from build123d import *

# Parameters (mm, degrees)
BOSS_EXTRU_1_DEPTH      = 11.3
ESQUISSE2_W             = 8.6
ESQUISSE2_H             = 11.3
BOSS_EXTRU_2_DEPTH      = 1
ESQUISSE8_W             = 11.3
ESQUISSE8_H             = 1
BOSS_EXTRU_5_DEPTH      = 10
ESQUISSE9_W             = 2
ESQUISSE9_H             = 11.3
BOSS_EXTRU_6_DEPTH      = 7.8
ESQUISSE10_W            = 11.3
ESQUISSE10_H            = 2
BOSS_EXTRU_7_DEPTH      = 39.7
ESQUISSE11_W            = 2
ESQUISSE11_H            = 11.3
BOSS_EXTRU_8_DEPTH      = 11.3
ESQUISSE12_W            = 2
ESQUISSE12_H            = 11.3
BOSS_EXTRU_9_DEPTH      = 11.3
BOSS_EXTRU_10_DEPTH     = 11.3
ESQUISSE14_W            = 1
ESQUISSE14_H            = 11.3
BOSS_EXTRU_11_DEPTH     = 5.8
ESQUISSE16_W            = 11.3
ESQUISSE16_H            = 6.8
ENL_V_MAT_EXTRU_1_DEPTH = 1
ESQUISSE19_R            = 2
ENL_V_MAT_EXTRU_3_DEPTH = 10


with BuildPart() as part:
    # Esquisse1 → Boss.-Extru.1 (new body)
    with BuildSketch(Plane.XY):
        Polygon((-20.6, 1), (-20.6, 0), (-24.6, 0), (-24.6, 13.6), (0, 13.6), (0, 0), (-4, 0), (-4, 1), (-1, 1), (-1, 12.6), (-23.6, 12.6), (-23.6, 1), align=None)
    extrude(amount=BOSS_EXTRU_1_DEPTH)

    # Esquisse2 → Boss.-Extru.2 (add)
    with BuildSketch(Plane(origin=(0, 13.6, 0), x_dir=(1, 0, 0), z_dir=(0, 1, 0))):
        with Locations((-12.3, -5.65)):
            Rectangle(ESQUISSE2_W, ESQUISSE2_H)
    extrude(amount=BOSS_EXTRU_2_DEPTH)

    # Esquisse8 → Boss.-Extru.5 (add)
    with BuildSketch(Plane(origin=(-8, 0, 0), x_dir=(0, 0, -1), z_dir=(1, 0, 0))):
        with Locations((-5.65, 14.1)):
            Rectangle(ESQUISSE8_W, ESQUISSE8_H)
    extrude(amount=BOSS_EXTRU_5_DEPTH)

    # Esquisse9 → Boss.-Extru.6 (add)
    with BuildSketch(Plane.XZ.offset(-13.6)):
        with Locations((1, 5.65)):
            Rectangle(ESQUISSE9_W, ESQUISSE9_H)
    extrude(amount=BOSS_EXTRU_6_DEPTH)

    # Esquisse10 → Boss.-Extru.7 (add)
    with BuildSketch(Plane(origin=(2, 0, 0), x_dir=(0, 0, -1), z_dir=(1, 0, 0))):
        with Locations((-5.65, 6.8)):
            Rectangle(ESQUISSE10_W, ESQUISSE10_H)
    extrude(amount=BOSS_EXTRU_7_DEPTH)

    # Esquisse11 → Boss.-Extru.8 (add)
    with BuildSketch(Plane.XZ.offset(-5.8)):
        with Locations((40.7, 5.65)):
            Rectangle(ESQUISSE11_W, ESQUISSE11_H)
    extrude(amount=BOSS_EXTRU_8_DEPTH)

    # Esquisse12 → Boss.-Extru.9 (add)
    with BuildSketch(Plane(origin=(0, 7.8, 0), x_dir=(1, 0, 0), z_dir=(0, 1, 0))):
        with Locations((40.7, -5.65)):
            Rectangle(ESQUISSE12_W, ESQUISSE12_H)
    extrude(amount=BOSS_EXTRU_9_DEPTH)

    # Esquisse13 → Boss.-Extru.10 (add)
    with BuildSketch(Plane.XY.offset(11.3)):
        Polygon((-16.6, 14.6), (-25.6, 14.6), (-25.6, 0), (-24.6, 0), (-24.6, 13.6), (-16.6, 13.6), align=None)
    extrude(amount=-BOSS_EXTRU_10_DEPTH)

    # Esquisse14 → Boss.-Extru.11 (add)
    with BuildSketch(Plane.XZ.offset(-5.8)):
        with Locations((0.5, 5.65)):
            Rectangle(ESQUISSE14_W, ESQUISSE14_H)
    extrude(amount=BOSS_EXTRU_11_DEPTH)

    # Esquisse16 → Enlèv. mat.-Extru.1 (cut)
    with BuildSketch(Plane(origin=(2, 0, 0), x_dir=(0, 0, -1), z_dir=(1, 0, 0))):
        with Locations((-5.65, 11.2)):
            Rectangle(ESQUISSE16_W, ESQUISSE16_H)
    extrude(amount=-ENL_V_MAT_EXTRU_1_DEPTH, mode=Mode.SUBTRACT)

    # Esquisse19 → Enlèv. mat.-Extru.3 (cut)
    with BuildSketch(Plane(origin=(41.7, 0, 0), x_dir=(0, 0, -1), z_dir=(1, 0, 0))):
        with Locations((-5.65, 13.45)):
            Circle(ESQUISSE19_R)
        with Locations((-5.65, 2.15)):
            Circle(ESQUISSE19_R)
    extrude(amount=-ENL_V_MAT_EXTRU_3_DEPTH, mode=Mode.SUBTRACT)


solid = part.part
Build history of the part. All positions in model axes, mm. A direction names the side the tool comes from. Coordinates: 2 decimals unless noted, no trailing zeros. Order: outer loops, then holes, each group sorted by start corner. A loop starts at its lowest first (then second) coordinate and runs counter-clockwise, first axis right, second up. Notation, with made-up numbers: (-3.5, 63.25) -> (11.5, 63.25) arc R20 cw to (11.5, 71.25) -> close; hole circle Ø6 at (-13.75, -3). An arc over 180 degrees is marked (long way). One line per item, written item: value.
(1) Tool access for faces 1 (the cylindrical face through (40.714, 1.384, 3.803)), 2 (the flat face through (-2, 0, 6)), 3 (the flat face through (20, 5.8, 6)), 4 (the flat face through (21, 7.8, 6)): list every direction of +Z, -Z, +X, -X, +Y, -Y with a clear straight run to the whole face (end or side of a thin tool).
Checked values:
face 1: +X
face 2: +Z, -Z, -X, -Y
face 3: +Z, -Z, -Y
face 4: +Z, -Z, +Y
(2) Slice it at C-C, the plane y = 13.45. List the corners of the cut face in (x, z), plus the area to 3 significant figures.
Checked values:
outline: (-25.6, 0) -> (1, 0) -> (1, 11.3) -> (-25.6, 11.3) -> close; (39.7, 0) -> (41.7, 0) -> (41.7, 3.65) -> (39.7, 3.65) -> close; (39.7, 7.65) -> (41.7, 7.65) -> (41.7, 11.3) -> (39.7, 11.3) -> close
area: 315 mm2
(3) Mould opens along X. For faces 5 (the flat face through (-22, 1, 6)), 6 (the flat face through (41.7, 7, 6)), 7 (the flat face through (-23, 0, 6)) say: pulls with the +X half, pulls with the -X half, needs draft (parallel to the pull), parting line crosses it, or undercut.
Checked values:
face 5: undercut
face 6: pulls with the +X half
face 7: needs draft
(4) Drop flat-ended pins along their axis: pin 1 Ø5.5 at (x, z) = (-23, 3) entering from -Y; pin 2 Ø4 at (x, z) = (-0.5, 3) entering from +Y; pin 3 Ø5.5 at (x, z) = (16.5, 7) entering from +Y. Give the stop position or say it passes through.
Checked values:
pin 1: y = 0
pin 2: y = 14.6
pin 3: y = 7.8
(5) Slice it at B-B, the plane y = 7. List the corners of the cut face in (x, z), plus the area to 3 significant figures.
Checked values:
outline: (-25.6, 0) -> (-23.6, 0) -> (-23.6, 11.3) -> (-25.6, 11.3) -> close; (-1, 0) -> (41.7, 0) -> (41.7, 11.3) -> (-1, 11.3) -> close
area: 505 mm2
(6) Slice it at A-A, the plane z = 5.65. List the corners of the cut face in (x, y), plus the area to 3 significant figures.
Checked values:
outline: (-25.6, 0) -> (-20.6, 0) -> (-20.6, 1) -> (-23.6, 1) -> (-23.6, 12.6) -> (-1, 12.6) -> (-1, 1) -> (-4, 1) -> (-4, 0) -> (1, 0) -> (1, 5.8) -> (39.7, 5.8) -> (39.7, 4.15) -> (41.7, 4.15) -> (41.7, 11.45) -> (39.7, 11.45) -> (39.7, 7.8) -> (1, 7.8) -> (1, 14.6) -> (-25.6, 14.6) -> close; (39.7, -5.5) -> (41.7, -5.5) -> (41.7, 0.15) -> (39.7, 0.15) -> close; (39.7, 15.45) -> (41.7, 15.45) -> (41.7, 19.1) -> (39.7, 19.1) -> close
area: 220 mm2
(7) Probe line 1 (X direction, y = 4.5, z = 9.5); line 2 (Y direction, x = 41.3, z = 5.65); line 3 (X direction, y = 13.5, z = 9.75). List the from-to ranges inside material, lowest first. Write a range as [from, to].
Checked values:
line 1: [-25.6, -23.6], [-1, 1], [39.7, 41.7]
line 2: [-5.5, 0.15], [4.15, 11.45], [15.45, 19.1]
line 3: [-25.6, 1], [39.7, 41.7]
(8) Slice it at D-D, the plane y = 2.15. List the corners of the cut face in (x, z), plus the area to 3 significant figures.
Checked values:
outline: (-25.6, 0) -> (-23.6, 0) -> (-23.6, 11.3) -> (-25.6, 11.3) -> close; (-1, 0) -> (1, 0) -> (1, 11.3) -> (-1, 11.3) -> close; (39.7, 0) -> (41.7, 0) -> (41.7, 3.65) -> (39.7, 3.65) -> close; (39.7, 7.65) -> (41.7, 7.65) -> (41.7, 11.3) -> (39.7, 11.3) -> close
area: 59.8 mm2
